Could you check a few things on this model? Use its own coordinates, in mm. A direction names the side the tool comes from. Coordinates: 2 decimals unless noted, no trailing zeros. Order: outer loops, then holes, each group sorted by start corner. A loop starts at its lowest first (then second) coordinate and runs counter-clockwise, first axis right, second up. Notation, with made-up numbers: (38.25, 37.5) -> (81.25, 37.5) arc R25 cw to (81.25, 64.5) -> close; hole circle Ø3 at (12.5, 20). An arc over 180 degrees is marked (long way). Use a Markdown table: item, result. Add a question column.
1) Thinking about a two-plate mould opening in Z: for faces 5 (the cylindrical face through (-68, 1, 0)), 6 (the flat face through (-73.79, 1, -1)), 7 (the cylindrical face through (-51.1, -13.6, 0.2)), which applies, +Z half, -Z half, draft (parallel to the pull), parting line (faces both ways), or undercut?
2) If I drill on L1, parallel to Y at x = -67.75, z = -4.5; L2, parallel to Y at x = -66, z = 0; L3, parallel to X at y = 2, z = 3.75, over which ranges is the centre line in solid material (lowest first)? Write a range as [from, to].
3) If we section it at A-A (x = -71): Write out the boundary of the cut face in (y, z).
4) If we section it at B-B (z = -11.5): Write out the boundary of the cut face in (x, y), plus the area to 3 significant figures.
5) Which directions (+Z, -Z, +X, -X, +Y, -Y) give clear straight access to the entire face, cutting with the end or side of a thin tool? Please do faces 1 (the cylindrical face through (-58.702, 13.058, -2.103)), 2 (the flat face through (-68.09, -2, 0)), 3 (the cylindrical face through (-37.06, -13.18, -2.93)), 4 (the cylindrical face through (-73.283, -0.481, -1.526)).
6) Will these pins go through, and if not, where does the flat tip stop? pin 1 Ø1.6 at (y, z) = (11.5, 0) entering from -X; pin 2 Ø0.5 at (x, y) = (-56.5, 12) entering from -Z; pin 3 Ø0.5 at (x, z) = (-57, -0.5) entering from -Y; pin 4 Ø1.5 at (x, y) = (-63.5, -5) entering from +Z.
7) If we section it at C-C (x = -51): Write out the boundary of the cut face in (y, z) (3 decimals).
8) If we section it at D-D (y = -9.5): Write out the boundary of the cut face in (x, z), plus the area to 3 significant figures.
```python
from build123d import *

# Parameters (mm, degrees)
PUMP_OD_SKETCH_R          = 13.5
PUMP_OD_EXTRUDE_DEPTH     = 31.2
PUMP_START                = 12.3
PUMP_MIDDLE_SKETCH_R      = 13.55
PUMP_MIDDLE_EXTRUDE_DEPTH = 12
DIAPHRAGM_START           = -3.6
DIAPHRAGM_EXTRUDE_DEPTH   = 1.3
SCREW_POCKET_CUT_DEPTH    = 6.9
SCREW_POCKET_FILLET_R     = 0.8
SCEW_HEAD_SKETCH_R        = 1.3
SCREW_HEAD_EXTRUDE_DEPTH  = 1.8
SCREW_HEAD_FILLET_R       = 1
SCREW_DRIVE_CUT_DEPTH     = 1
WASHER_SKETCH_R           = 1.581796131
WASHER_EXTRUDE_DEPTH      = 0.4
NOZZLE_LPATTERN_COUNT     = 2
NOZZLE_LPATTERN_PITCH     = 9


with BuildPart() as part:
    # Pump OD Sketch → Pump OD Extrude (new body)
    with BuildSketch(Plane.ZY.offset(31)):
        Circle(PUMP_OD_SKETCH_R)
    extrude(amount=PUMP_OD_EXTRUDE_DEPTH)

    # Pump Middle Sketch → Pump Middle Extrude (add)
    with BuildSketch(Plane.ZY.offset(31).offset(PUMP_START)):
        Circle(PUMP_MIDDLE_SKETCH_R)
    extrude(amount=PUMP_MIDDLE_EXTRUDE_DEPTH)

    # Diaphragm Sketch → Diaphragm Extrude (add)
    with BuildSketch(Plane.ZY.offset(55.3).offset(DIAPHRAGM_START)):
        with BuildLine():
            Line((-1.825, 12.291819434), (1.825, 12.291819434))
            Line((1.825, 12.291819434), (1.825, 13.408145845))
            ThreePointArc((1.825, 13.408145845), (1.845637465, 13.453429295), (1.893353028, 13.467561558))
            ThreePointArc((1.893353028, 13.467561558), (11.777945491, 6.8), (12.60992695, -5.094088958))
            ThreePointArc((12.60992695, -5.094088958), (12.57383027, -5.128345717), (12.524294919, -5.123576561))
            Line((12.524294919, -5.123576561), (11.557527888, -4.565413355))
            Line((11.557527888, -4.565413355), (9.732527888, -7.726406079))
            Line((9.732527888, -7.726406079), (10.699294919, -8.284569284))
            ThreePointArc((10.699294919, -8.284569284), (10.728192805, -8.325083578), (10.716573922, -8.373472599))
            ThreePointArc((10.716573922, -8.373472599), (0, -13.6), (-10.716573922, -8.373472599))
            ThreePointArc((-10.716573922, -8.373472599), (-10.728192805, -8.325083578), (-10.699294919, -8.284569284))
            Line((-10.699294919, -8.284569284), (-9.732527888, -7.726406079))
            Line((-9.732527888, -7.726406079), (-11.557527888, -4.565413355))
            Line((-11.557527888, -4.565413355), (-12.524294919, -5.123576561))
            ThreePointArc((-12.524294919, -5.123576561), (-12.57383027, -5.128345717), (-12.60992695, -5.094088958))
            ThreePointArc((-12.60992695, -5.094088958), (-11.777945491, 6.8), (-1.893353028, 13.467561558))
            ThreePointArc((-1.893353028, 13.467561558), (-1.845637465, 13.453429295), (-1.825, 13.408145845))
            Line((-1.825, 13.408145845), (-1.825, 12.291819434))
        make_face()
    extrude(amount=-DIAPHRAGM_EXTRUDE_DEPTH)

    # Screw Pocket Sketch → Screw Pocket Cut (cut)
    with BuildSketch(Plane.ZY.offset(62.2)):
        with BuildLine():
            Line((-1.8, 11.6), (-1.8, 15.537585437))
            Line((-1.8, 15.537585437), (1.8, 15.537585437))
            Line((1.8, 15.537585437), (1.8, 11.6))
            ThreePointArc((1.8, 11.6), (0, 9.8), (-1.8, 11.6))
        make_face()
    extrude(amount=-SCREW_POCKET_CUT_DEPTH, mode=Mode.SUBTRACT)

    # Screw Pocket Fillet
    screw_pocket_fillet_edges = [part.edges().sort_by_distance(p)[0] for p in [
        (-58.75, 13.379461873, -1.8),
        (-58.75, 13.379461873, 1.8),
    ]]
    fillet(screw_pocket_fillet_edges, radius=SCREW_POCKET_FILLET_R)

    # Scew Head Sketch → Screw Head Extrude (add)
    with BuildSketch(Plane.ZY.offset(55.3)):
        with Locations((0, 11.6)):
            Circle(SCEW_HEAD_SKETCH_R)
    extrude(amount=SCREW_HEAD_EXTRUDE_DEPTH)

    # Screw Head Fillet
    screw_head_fillet_edges = [part.edges().sort_by_distance(p)[0] for p in [
        (-57.1, 11.6, -1.3),
    ]]
    fillet(screw_head_fillet_edges, radius=SCREW_HEAD_FILLET_R)

    # Sketch10 → Screw Drive Cut (cut)
    with BuildSketch(Plane.ZY.offset(57.1)):
        Polygon((0.15, 11.75), (0.15, 12.4), (-0.15, 12.4), (-0.15, 11.75), (-0.8, 11.75), (-0.8, 11.45), (-0.15, 11.45), (-0.15, 10.8), (0.15, 10.8), (0.15, 11.45), (0.8, 11.45), (0.8, 11.75), align=None)
    extrude(amount=-SCREW_DRIVE_CUT_DEPTH, mode=Mode.SUBTRACT)

    # Washer Sketch → Washer Extrude (add)
    with BuildSketch(Plane.ZY.offset(55.3)):
        with Locations((0, 11.6)):
            Circle(WASHER_SKETCH_R)
    extrude(amount=WASHER_EXTRUDE_DEPTH)

    # Center Nozzle Sketch → Center Nozzle Revolve (revolve)
    with BuildSketch(Plane.XY, mode=Mode.PRIVATE) as center_nozzle_revolve_sk:
        Polygon((-73.789716671, 1.6), (-72.789716671, 1.6), (-68.089716671, 2.4), (-68.089716671, 1.8), (-65.2, 1.8), (-62.2, 2.7), (-62.2, 1), (-73.789716671, 1), align=None)
    center_nozzle_revolve = revolve(center_nozzle_revolve_sk.sketch.rotate(Axis((0, 0, 0), (-1, 0, 0)), 90), axis=Axis((0, 0, 0), (-1, 0, 0)))

    # Nozzle LPattern: Center Nozzle Revolve ×2
    with Locations(*[Vector(0, 0.8660254037844379, -0.5000000000000012) * (i * NOZZLE_LPATTERN_PITCH) for i in range(1, NOZZLE_LPATTERN_COUNT)]):
        add(center_nozzle_revolve)


solid = part.part
```
Answer sheet:
| question | item | result |
|---|---|---|
| 1 | face 5 | undercut |
| 1 | face 6 | draft |
| 1 | face 7 | parting line |
| 2 | L1 | [5.99, 6.79], [8.79, 9.59] |
| 2 | L2 | [-1.8, -1], [1, 1.8] |
| 2 | L3 | [-62.2, -31] |
| 3 | outline | circle Ø3.81 at (0, 0); circle Ø3.81 at (7.79, -4.5); hole circle Ø2 at (0, 0); hole circle Ø2 at (7.79, -4.5) |
| 4 | outline | (-62.2, -7.07) -> (-55.3, -7.07) -> (-55.3, -7.17) -> (-43.3, -7.17) -> (-43.3, -7.07) -> (-31, -7.07) -> (-31, 7.07) -> (-43.3, 7.07) -> (-43.3, 7.17) -> (-50.4, 7.17) -> (-50.4, 7.26) -> (-51.7, 7.26) -> (-51.7, 7.17) -> (-55.3, 7.17) -> (-55.3, 7.07) -> (-62.2, 7.07) -> close |
| 4 | area | 444 mm2 |
| 5 | face 1 | -X, +Y |
| 5 | face 2 | none |
| 5 | face 3 | +X |
| 5 | face 4 | -X |
| 6 | pin 1 | x = -57.1 |
| 6 | pin 2 | z = -6.65 |
| 6 | pin 3 | y = -13.5 |
| 6 | pin 4 | through |
| 7 | outline | (-8.373, -10.717) arc R0.06 ccw to (-8.296, -10.714) arc R13.55 ccw to (-5.13, -12.541) arc R0.06 ccw to (-5.094, -12.61) arc R13.6 ccw to (13.468, -1.893) arc R0.06 ccw to (13.426, -1.828) arc R13.55 ccw to (13.426, 1.828) arc R0.06 ccw to (13.468, 1.893) arc R13.6 ccw to (-5.094, 12.61) arc R0.06 ccw to (-5.13, 12.541) arc R13.55 ccw to (-8.296, 10.714) arc R0.06 ccw to (-8.373, 10.717) arc R13.6 ccw to start |
| 8 | outline | (-62.2, -9.59) -> (-55.3, -9.59) -> (-55.3, -9.66) -> (-51.7, -9.66) -> (-51.7, -9.73) -> (-50.4, -9.73) -> (-50.4, -9.66) -> (-43.3, -9.66) -> (-43.3, -9.59) -> (-31, -9.59) -> (-31, 9.59) -> (-43.3, 9.59) -> (-43.3, 9.66) -> (-50.4, 9.66) -> (-50.4, 9.73) -> (-51.7, 9.73) -> (-51.7, 9.66) -> (-55.3, 9.66) -> (-55.3, 9.59) -> (-62.2, 9.59) -> close |
| 8 | area | 600 mm2 |
